```python
from build123d import *

# Parameters (mm, degrees)
SKETCH2_W               = 12.7
SKETCH2_H               = 38.1
SKETCH2_R               = 3.175
BOSS_EXTRUDE1_DEPTH     = 9.525
SKETCH3_R               = 4.699
BOSS_EXTRUDE2_DEPTH     = 9.525
SKETCH6_W               = 6.35
SKETCH6_H               = 44.45
BOSS_EXTRUDE3_DEPTH     = 25.4
FILLET1_R               = 6.35
FILLET4_R               = 3.175
CUT_EXTRUDE1_DEPTH      = 72.278573361
CUT_EXTRUDE1_DEPTH_BACK = 3.175
SKETCH8_R               = 1.004
CUT_EXTRUDE2_DEPTH      = 72.278573361
SKETCH9_R               = 1.726999975
CUT_EXTRUDE3_DEPTH      = 71.781852519


with BuildPart() as part:
    # Sketch2 → Boss-Extrude1 (new body)
    with BuildSketch(Plane(origin=(0, 0, 0), x_dir=(0, 0, -1), z_dir=(1, 0, 0))):
        Rectangle(SKETCH2_W, SKETCH2_H)
        with Locations(Location((0, 0, 0), (0, 0, 180))):
            Circle(SKETCH2_R, mode=Mode.SUBTRACT)
    extrude(amount=BOSS_EXTRUDE1_DEPTH)

    # Sketch3 → Boss-Extrude2 (add)
    with BuildSketch(Plane.ZY):
        with Locations(Location((0, 0, 0), (0, 0, 180))):
            Circle(SKETCH3_R)
    extrude(amount=BOSS_EXTRUDE2_DEPTH)

    # Sketch6 → Boss-Extrude3 (add, symmetric)
    with BuildSketch(Plane(origin=(3.175, 0, 0), x_dir=(0, 0, -1), z_dir=(1, 0, 0))):
        with Locations((3.175, 41.275)):
            Rectangle(SKETCH6_W, SKETCH6_H)
    extrude(amount=BOSS_EXTRUDE3_DEPTH, both=True)

    # Fillet1
    fillet1_edges = [part.edges().sort_by_distance(p)[0] for p in [
        (4.7625, 19.05, 0),
    ]]
    fillet(fillet1_edges, radius=FILLET1_R - 0.0001)  # a hair under: the kernel refuses the full size

    # Fillet4
    fillet4_edges = [part.edges().sort_by_distance(p)[0] for p in [
        (9.525, 22.22495, 0),
        (0, 22.22495, 0),
        (0, 19.05, -3.175),
        (9.525, 19.05, -3.175),
    ]]
    fillet(fillet4_edges, radius=FILLET4_R)

    # Sketch7 → Cut-Extrude1 (cut, two sides: drawn at the far end of the back side and taken through both)
    with BuildSketch(Plane(origin=(9.525, 0, 0), x_dir=(0, 0, -1), z_dir=(1, 0, 0)).offset(-CUT_EXTRUDE1_DEPTH_BACK)):
        with BuildLine():
            Line((2.595150061, -16.907830377), (4.619750173, -4.024678621))
            ThreePointArc((4.619750173, -4.024678621), (6.127000091, 2.2e-08), (4.619750173, 4.024678665))
            Line((4.619750173, 4.024678665), (2.595150061, 16.907830421))
            ThreePointArc((2.595150061, 16.907830421), (9.1e-08, 19.127000022), (-2.595149879, 16.907830421))
            Line((-2.595149879, 16.907830421), (-4.619749991, 4.024678665))
            ThreePointArc((-4.619749991, 4.024678665), (-6.126999909, 2.2e-08), (-4.619749991, -4.024678621))
            Line((-4.619749991, -4.024678621), (-2.595149879, -16.907830377))
            ThreePointArc((-2.595149879, -16.907830377), (9.1e-08, -19.126999978), (2.595150061, -16.907830377))
        make_face()
    extrude(amount=CUT_EXTRUDE1_DEPTH + CUT_EXTRUDE1_DEPTH_BACK, mode=Mode.SUBTRACT)

    # Sketch8 → Cut-Extrude2 (cut, through all)
    with BuildSketch(Plane(origin=(9.525, 0, 0), x_dir=(0, 0, -1), z_dir=(1, 0, 0))):
        with Locations((9.1e-08, -15.999999978)):
            Circle(SKETCH8_R)
        with Locations((9.1e-08, -12.999999978)):
            Circle(SKETCH8_R)
        with Locations((9.1e-08, -9.999999978)):
            Circle(SKETCH8_R)
        with Locations((9.1e-08, -6.999999978)):
            Circle(SKETCH8_R)
        with Locations((9.1e-08, 16.000000022)):
            Circle(SKETCH8_R)
        with Locations((9.1e-08, 13.000000022)):
            Circle(SKETCH8_R)
        with Locations((9.1e-08, 10.000000022)):
            Circle(SKETCH8_R)
        with Locations((9.1e-08, 7.000000022)):
            Circle(SKETCH8_R)
    extrude(amount=-CUT_EXTRUDE2_DEPTH, mode=Mode.SUBTRACT)

    # Sketch9 → Cut-Extrude3 (cut, through all)
    with BuildSketch(Plane(origin=(0, 0, -6.35), x_dir=(-1, 0, 0), z_dir=(0, 0, -1))):
        with Locations((-22.225, 57.15)):
            Circle(SKETCH9_R)
        with Locations((15.875, 57.15)):
            Circle(SKETCH9_R)
        with Locations((17.839802872, 25.4)):
            Circle(SKETCH9_R)
        with Locations((-22.225, 25.4)):
            Circle(SKETCH9_R)
    extrude(amount=-CUT_EXTRUDE3_DEPTH, mode=Mode.SUBTRACT)


solid = part.part
```
Here's how the part is built. I have some questions about the finished solid (model axes, mm). A direction names the side the tool comes from. Coordinates: 2 decimals unless noted, no trailing zeros. Loops run counter-clockwise (first coordinate to the right, second up) from the corner with the lowest first, then second, coordinate; pieces in that order, holes last. Notation, with made-up numbers: M 58.5,-32 L 100.5,-32 A18 ccw 100.5,-1 Z; hole C 37,-4 d8. An arc over 180 degrees is marked long. One line per item, written item: value.
1. On a 3-axis mill with a long thin cutter (end or side, diameter ignored), from which of +Z, -Z, +X, -X, +Y, -Y can I reach the whole of each face in a straight line? I mean faces 5 (the flat face through (-9.525, 0, 0)), 6 (the cylindrical face through (-4.7, -4.66, 0.61)), 7 (the flat face through (8, 10.38, -3.62)). Say none if no direction works.
Geometry says:
face 5: +Z, -Z, -X, -Y
face 6: -X
face 7: +X
2. Imagine slicing it at D-D (x = -1.5). List the corners of the cut face in (y, z) for me, and give its area (3 significant figures).
Geometry says:
outline: C 0,0 d9.4; M 18.57,-6.35 L 63.5,-6.35 L 63.5,0 L 25.4,0 A6.35 cw 22.98,0.48 L 18.57,0.48 Z
area: 357 mm2
3. Imagine slicing it at C-C (y = 10). List the corners of the cut face in (x, z) for me (3 decimals), and give its area (3 significant figures).
Geometry says:
outline: M 0,-6.35 L 9.525,-6.35 L 9.525,-3.681 L 6.35,-3.681 L 6.35,-1.004 L 0,-1.004 Z; M 0,1.004 L 6.35,1.004 L 6.35,3.681 L 9.525,3.681 L 9.525,6.35 L 0,6.35 Z
area: 84.8 mm2
4. Imagine slicing it at A-A (y = 57.15). List the corners of the cut face in (x, z) for me (3 decimals).
Geometry says:
outline: M -22.225,-6.35 L -17.602,-6.35 L -17.602,0 L -22.225,0 Z; M -14.148,-6.35 L 20.498,-6.35 L 20.498,0 L -14.148,0 Z; M 23.952,-6.35 L 28.575,-6.35 L 28.575,0 L 23.952,0 Z
5. Please list where these lines run through material, in increasing order: probe 1 along X at (y, z) = (12, 1.25); probe 2 along Z at (x, y) = (-13.5, 26); probe 3 along Y at (x, z) = (16, -2.5).
Geometry says:
probe 1: x = 0 to 6.35
probe 2: z = -6.35 to 0
probe 3: y = 19.05 to 63.5
6. Will these pins go through, and if not, where does the flat tip stop? pin 1 Ø1.5 at (y, z) = (1, -1.5) entering from +X; pin 2 Ø4 at (x, z) = (-7.5, -4) entering from -Y; pin 3 Ø7.5 at (y, z) = (0, 0) entering from +X.
Geometry says:
pin 1: stops at x = 0
pin 2: stops at y = -4.25
pin 3: stops at x = 6.35
7. Thinking about a two-plate mould opening in Y: for faces 1 (the cylindrical face through (10.43, 18.095, -4.166)), 2 (the flat face through (9.525, -5, -5)), 3 (the flat face through (-13, 19.05, -3)), 4 (the cylindrical face through (4.874, 21.815, 1.109)), which applies, +Y half, -Y half, draft (parallel to the pull), parting line (faces both ways), or undercut?
Geometry says:
face 1: -Y half
face 2: draft
face 3: undercut
face 4: +Y half
